Could you check a few things on this drawing? It's one solid part, dimensions in mm from its lowest x, y, z. A direction names the side the tool comes from. Give positions to 0.01 mm unless a question says otherwise; leave off trailing zeros. Loops run counter-clockwise (first coordinate to the right, second up) from the corner with the lowest first, then second, coordinate; pieces in that order, holes last.
Q1. Suppose I cut it at B-B (y = 1.5). List the corners of the cut face in (x, z) for me.
Q2. Thinking about a two-plate mould opening in Y: for the marked faces 1, 2, 3 and 4, which applies, pulls with the +Y half, pulls with the -Y half, needs draft (parallel to the pull), parting line crosses it, or undercut?
Q3. I'm going to push flat-ended pins straight in: P1, Ø1.8, axis at x = 5.5, z = 28.5, coming from the +Y side; P2, Ø1, axis at x = 9, y = 5.5, coming from the +Z side. Where does each tip first touch, or does it pass through?
Q4. Suppose I cut it at A-A (x = 6). List the corners of the cut face in (y, z) for me, and give its area (3 significant figures).
Q5. Suppose I cut it at C-C (y = 4). List the corners of the cut face in (x, z) for me, and give its area (3 significant figures).
Q6. Suppose I cut it at D-D (z = 21). List the corners of the cut face in (x, y) for me, and give its area (3 significant figures).
Q7. I need wall thicknesses on probe 1 along Z at (x, y) = (6.75, 9.25); probe 2 along Y at (x, z) = (1.5, 20); probe 3 along Y at (x, z) = (1.5, 23.55). Which ranges of each line are inside material? Lowest first, please.
Q8. For the marked faces 5, 6 and 7, which set-ups out of +Z, -Z, +X, -X, +Y, -Y let a thin tool reach every point of the face, with its end or its side?
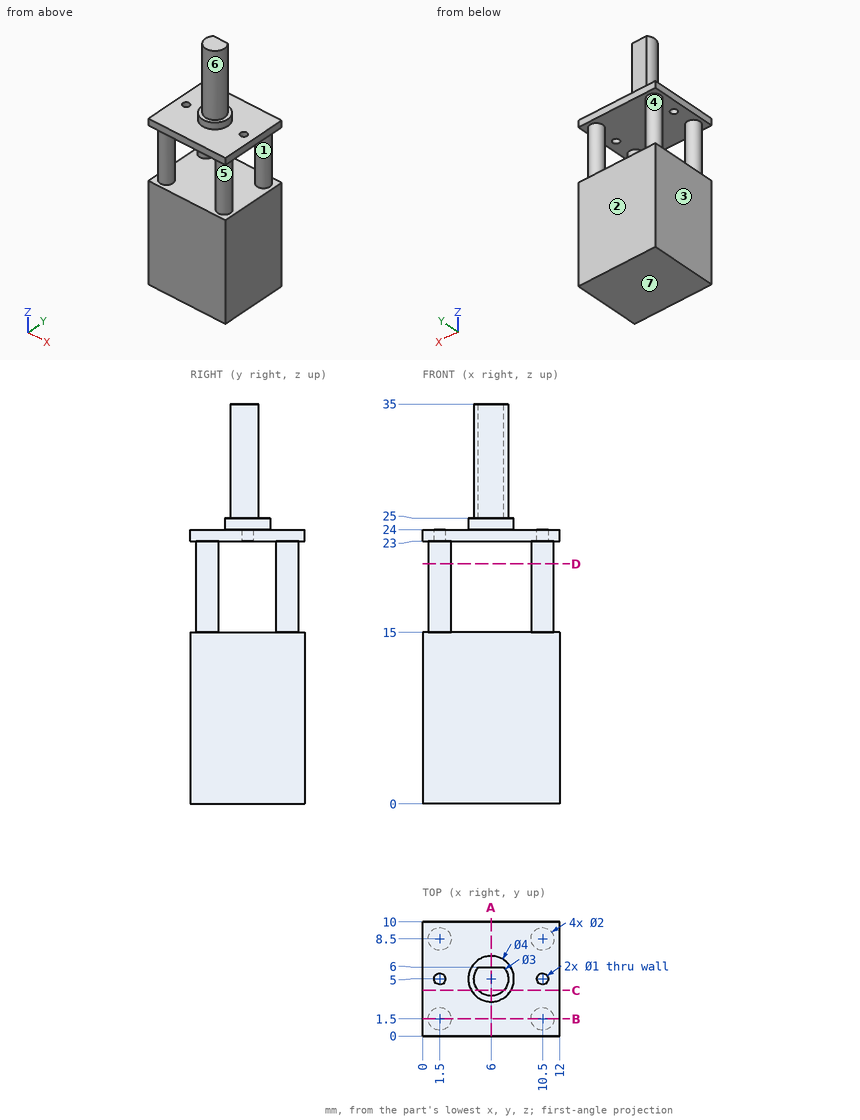
Solutions:
1. outline: (0, 0) - (12, 0) - (12, 15) - (11.5, 15) - (11.5, 23) - (12, 23) - (12, 24) - (0, 24) - (0, 23) - (0.5, 23) - (0.5, 15) - (0, 15) - close; hole (2.5, 15) - (9.5, 15) - (9.5, 23) - (2.5, 23) - close
2. face 1: undercut
2. face 2: pulls with the +Y half
2. face 3: needs draft
2. face 4: undercut
3. P1: stops at y = 6
3. P2: stops at z = 24
4. outline: (0, 0) - (10, 0) - (10, 15) - (0, 15) - close; (0, 23) - (10, 23) - (10, 24) - (7, 24) - (7, 25) - (6, 25) - (6, 35) - (3.5, 35) - (3.5, 25) - (3, 25) - (3, 24) - (0, 24) - close
4. area: 189 mm2
5. outline: (0, 0) - (12, 0) - (12, 15) - (0, 15) - close; (0, 23) - (12, 23) - (12, 24) - (7.73, 24) - (7.73, 25) - (7.12, 25) - (7.12, 35) - (4.88, 35) - (4.88, 25) - (4.27, 25) - (4.27, 24) - (0, 24) - close
5. area: 218 mm2
6. outline: circle Ø2 at (1.5, 1.5); circle Ø2 at (1.5, 8.5); circle Ø2 at (10.5, 1.5); circle Ø2 at (10.5, 8.5)
6. area: 12.6 mm2
7. probe 1: z = 0 to 15, 23 to 24
7. probe 2: y = 0.5 to 2.5, 7.5 to 9.5
7. probe 3: y = 0 to 4.5, 5.5 to 10
8. face 5: none
8. face 6: +Z
8. face 7: -Z, +X, -X, +Y, -Y
